Geometry check sheet. Reference: the model listing, model coordinates, mm. A direction names the side the tool comes from. Give positions to 0.01 mm unless a question says otherwise; leave off trailing zeros. Write each loop counter-clockwise with the first axis right and the second up, starting at its lowest first coordinate (ties: lowest second). Pieces come first, ordered by that corner, then holes.
(1) Cross-section at A-A (x = 0). Record the boundary of the cut face in (y, z), and give its area (3 significant figures).
(2) Cross-section at D-D (x = 28.5). Record the boundary of the cut face in (y, z).
(3) Thickness scan on line 1 along Y through (x, z) = (6.5, -7); line 2 along X through (y, z) = (32.6, 35); line 3 along X through (y, z) = (29, -26). Record the ranges inside material, lowest first.
(4) Cross-section at B-B (z = 35). Record the boundary of the cut face in (x, y).
(5) Depth check by flat-ended pin: P1, Ø11, axis at x = 6.5, y = 43, coming from the +Z side; P2, Ø4, axis at x = -17, z = 71.5, coming from the -Y side; P3, Ø4, axis at y = 12.5, z = 72, coming from the +X side; P4, Ø8, axis at x = -79.5, z = 12.5, coming from the -Y side. Enter the tip coordinate at first touch or a pass-through.
(6) Mould release check, pull along Z, two halves, no side actions. Record for faces 1 (the flat face through (81.1, 24.65, 22.32)), 2 (the flat face through (-62.5, 14, 73)), 3 (the cylindrical face through (0.572, 33.042, 22.013)): +Z half, -Z half, draft (parallel to the pull), parting line (faces both ways), or undercut.
(7) Cross-section at C-C (y = 12.5). Record the boundary of the cut face in (x, z), and give its area (3 significant figures).
(8) Tool access check on faces 4 (the flat face through (21, 43, 35)), 5 (the flat face through (73.89, 14.79, 21.48)), 6 (the flat face through (-1, 28, 73)), 7 (the cylindrical face through (1.75, 43.986, 69.297)). Record the directions out of +Z, -Z, +X, -X, +Y, -Y that give a thin tool (end or side, any length) a straight path to the whole face; none if there is none.
```python
from build123d import *

# Parameters (mm, degrees)
AUFSATZ_LINEAR_AUSTRAGEN1_DEPTH = 50
SKIZZE2_W                       = 125
SKIZZE2_H                       = 28
SCHNITT_LINEAR_AUSTRAGEN1_DEPTH = 30
SCHNITT_LINEAR_AUSTRAGEN2_DEPTH = 30
SKIZZE4_R                       = 13
SCHNITT_LINEAR_AUSTRAGEN3_DEPTH = 30
SKIZZE5_W                       = 42
SKIZZE5_H                       = 42
SCHNITT_LINEAR_AUSTRAGEN4_DEPTH = 14
VERRUNDUNG1_R                   = 20


with BuildPart() as part:
    # Skizze1 → Aufsatz-Linear austragen1 (new body)
    with BuildSketch(Plane(origin=(0, 0, 0), x_dir=(1, 0, 0), z_dir=(0, 1, 0))):
        with BuildLine():
            ThreePointArc((-38.41106398, 28.906723224), (0, 46.897503241), (38.41106398, 28.906723224))
            Line((38.41106398, 28.906723224), (125, -75))
            Line((125, -75), (-125, -75))
            Line((-125, -75), (-38.41106398, 28.906723224))
        make_face()
    extrude(amount=AUFSATZ_LINEAR_AUSTRAGEN1_DEPTH)

    # Skizze2 → Schnitt-Linear austragen1 (cut)
    with BuildSketch(Plane.XY.offset(75)):
        with Locations((0, 14)):
            Rectangle(SKIZZE2_W, SKIZZE2_H)
    extrude(amount=-SCHNITT_LINEAR_AUSTRAGEN1_DEPTH, mode=Mode.SUBTRACT)

    # Skizze3 → Schnitt-Linear austragen2 (cut)
    with BuildSketch(Plane.XZ):
        with BuildLine():
            Line((114.324791937, 70), (-114.324791937, 70))
            Line((-114.324791937, 70), (-34.569957582, -25.705801226))
            ThreePointArc((-34.569957582, -25.705801226), (0, -41.897503241), (34.569957582, -25.705801226))
            Line((34.569957582, -25.705801226), (114.324791937, 70))
        make_face()
    extrude(amount=-SCHNITT_LINEAR_AUSTRAGEN2_DEPTH, mode=Mode.SUBTRACT)

    # Skizze4 → Schnitt-Linear austragen3 (cut)
    with BuildSketch(Plane(origin=(0, 50, 0), x_dir=(1, 0, 0), z_dir=(0, 1, 0))):
        with Locations(Location((0, -35, 0), (0, 0, 270))):
            Circle(SKIZZE4_R)
    extrude(amount=-SCHNITT_LINEAR_AUSTRAGEN3_DEPTH, mode=Mode.SUBTRACT)

    # Skizze5 → Schnitt-Linear austragen4 (cut)
    with BuildSketch(Plane(origin=(0, 50, 0), x_dir=(1, 0, 0), z_dir=(0, 1, 0))):
        with Locations((0, -35)):
            Rectangle(SKIZZE5_W, SKIZZE5_H)
    extrude(amount=-SCHNITT_LINEAR_AUSTRAGEN4_DEPTH, mode=Mode.SUBTRACT)

    # Verrundung1
    # the kernel refuses this fillet: 20 mm, written as the material it takes off along each edge
    with BuildSketch(Plane(origin=(175, 50, 75), x_dir=(0, -1, 0), z_dir=(-1, 0, 0))) as verrundung1_piece_1:
        with BuildLine():
            CenterArc((VERRUNDUNG1_R, -VERRUNDUNG1_R), VERRUNDUNG1_R, 90, 90)
            Line((0, -VERRUNDUNG1_R), (0, 0))
            Line((0, 0), (VERRUNDUNG1_R, 0))
        make_face()
    extrude(amount=350, mode=Mode.SUBTRACT)


solid = part.part
```
Reply:
1. outline: (0, -46.9) - (50, -46.9) - (50, 14) - (36, 14) - (36, 22) - (30, 22) - (30, -41.9) - (0, -41.9) - close; (28, 70) - (30, 70) - (30, 48) - (36, 48) - (36, 56) - (49.97, 56) arc R20 ccw to (30, 75) - (28, 75) - close
1. area: 1,770 mm2
2. outline: (0, -37.98) - (50, -37.98) - (50, 55) arc R20 ccw to (30, 75) - (28, 75) - (28, 70) - (30, 70) - (30, -31.72) - (0, -31.72) - close
3. line 1: y = 30 to 50
3. line 2: x = -91.67 to -13, 13 to 91.67
3. line 3: x = -40.83 to -34.32, 34.32 to 40.83
4. outline: (-91.67, 0) - (-85.16, 0) - (-85.16, 30) - (-13, 30) - (-13, 36) - (-21, 36) - (-21, 50) - (-91.67, 50) - close; (13, 30) - (85.16, 30) - (85.16, 0) - (91.67, 0) - (91.67, 50) - (21, 50) - (21, 36) - (13, 36) - close
5. P1: stops at z = 73.54
5. P2: stops at y = 28
5. P3: stops at x = 124.17
5. P4: passes through
6. face 1: -Z half
6. face 2: draft
6. face 3: undercut
7. outline: (-125, 75) - (-38.41, -28.91) arc R50 ccw to (38.41, -28.91) - (125, 75) - (62.5, 75) - (62.5, 70) - (114.32, 70) - (34.57, -25.71) arc R45 cw to (-34.57, -25.71) - (-114.32, 70) - (-62.5, 70) - (-62.5, 75) - close
7. area: 2,290 mm2
8. face 4: +Y
8. face 5: -Y
8. face 6: +Z, -Y
8. face 7: +Z, +X, -X, +Y
